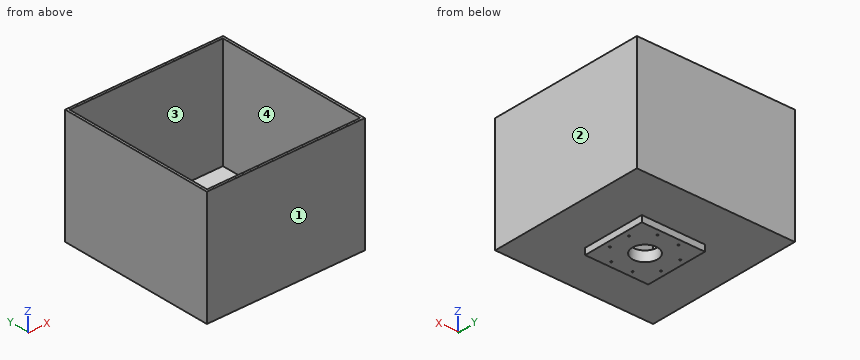
from build123d import *

# Parameters (mm, degrees)
F0_W     = 635
F0_H     = 635
F1_DEPTH = 15.875
F3_DEPTH = 447.675
F4_R     = 50.8
F5_DEPTH = 25.4
F6_W     = 254
F6_H     = 254
F6_R     = 3.4000059
F6_R_2   = 50.8
F7_DEPTH = 25.4


with BuildPart() as f1:
    # F0 (on Top) → F1 (new body)
    with BuildSketch(Plane.XY):
        with Locations((317.5, 317.5)):
            Rectangle(F0_W, F0_H)
    extrude(amount=F1_DEPTH)

    # F2 (on face) → F3 (join)
    with BuildSketch(Plane.XY.offset(15.875)):
        Polygon((0, 635), (0, 625.475), (9.525, 625.475), (625.475, 625.475), (625.475, 635), align=None)
        Polygon((0, 625.475), (0, 0), (9.525, 0), (9.525, 9.525), (9.525, 625.475), align=None)
        Polygon((9.525, 9.525), (9.525, 0), (635, 0), (635, 9.525), (625.475, 9.525), align=None)
        Polygon((625.475, 625.475), (625.475, 9.525), (635, 9.525), (635, 635), (625.475, 635), align=None)
    extrude(amount=F3_DEPTH)

    # F4 (on face) → F5 (cut, symmetric)
    with BuildSketch(Plane(origin=(0, 0, 0), x_dir=(1, 0, 0), z_dir=(0, 0, -1))):
        with Locations((317.5, -317.5)):
            Circle(F4_R)
    extrude(amount=F5_DEPTH, both=True, mode=Mode.SUBTRACT)

    # F6 (on face) → F7 (join)
    with BuildSketch(Plane(origin=(0, 0, 0), x_dir=(1, 0, 0), z_dir=(0, 0, -1))):
        with Locations((317.5, -317.5)):
            Rectangle(F6_W, F6_H)
        with Locations((274.7312995989, -420.7527765535)):
            Circle(F6_R, mode=Mode.SUBTRACT)
        with Locations((214.2472234465, -360.2687004011)):
            Circle(F6_R, mode=Mode.SUBTRACT)
        with Locations((360.2687004011, -420.7527765535)):
            Circle(F6_R, mode=Mode.SUBTRACT)
        with Locations((420.7527765535, -360.2687004011)):
            Circle(F6_R, mode=Mode.SUBTRACT)
        with Locations((214.2472234465, -274.7312995989)):
            Circle(F6_R, mode=Mode.SUBTRACT)
        with BuildLine():
            ThreePointArc((271.3312936989, -214.2472234465), (274.7312995989, -210.8472175465), (278.1313054989, -214.2472234465))
            ThreePointArc((278.1313054989, -214.2472234465), (274.7312995989, -217.6472293465), (271.3312936989, -214.2472234465))
        make_face(mode=Mode.SUBTRACT)
        with Locations((317.5, -317.5)):
            Circle(F6_R_2, mode=Mode.SUBTRACT)
        with Locations((420.7527765535, -274.7312995989)):
            Circle(F6_R, mode=Mode.SUBTRACT)
        with BuildLine():
            ThreePointArc((356.8686945011, -214.2472234465), (360.2687004011, -210.8472175465), (363.6687063011, -214.2472234465))
            ThreePointArc((363.6687063011, -214.2472234465), (360.2687004011, -217.6472293465), (356.8686945011, -214.2472234465))
        make_face(mode=Mode.SUBTRACT)
    extrude(amount=F7_DEPTH)


solid = f1.part
CAD build for the part. Positions are in the model's coordinates, mm. Face numbers are marked on the shaded views. Round coordinates to 2 decimals unless told otherwise and drop trailing zeros. Write each loop counter-clockwise with the first axis right and the second up, starting at its lowest first coordinate (ties: lowest second). Pieces come first, ordered by that corner, then holes. Notation, with made-up numbers: M 12.5,50 L 35.5,50 A7 cw 35.5,56 Z; hole C 39.25,55.5 d4. An arc over 180 degrees is marked long. Put each result on its own line as item: value. Start each with the question number.
1) Saw through at B-B, the plane z = 262. Write the cut outline in (x, y) (3 decimals), and give its area (3 significant figures).
2) Pin check, flat tips, straight feed: pin 1 Ø7.5 at (x, y) = (420, 360.5) entering from -Z; pin 2 Ø1.5 at (x, y) = (236, 336.5) entering from +Z (3 decimals); pin 3 Ø1.5 at (x, y) = (486.5, 170.5) entering from -Z. Stop position of each tip, or through.
3) Saw through at D-D, the plane y = 530. Write the cut outline in (x, z) (3 decimals).
4) Pull direction Y, two halves, no side cores. Call the marked faces 1, 2, 3 and 4: pulls with the +Y half, pulls with the -Y half, needs draft (parallel to the pull), parting line crosses it, or undercut.
5) Drill centre lines: probe 1 along X at (y, z) = (74, 62) (3 decimals); probe 2 along Z at (x, y) = (81, 546.5) (3 decimals). Where is each one in solid material? Low to high. Write a range as [from, to].
6) Saw through at A-A, the plane y = 317.5. Write the cut outline in (x, z) (3 decimals).
Resolved:
1. outline: M 0,0 L 635,0 L 635,635 L 0,635 Z; hole M 9.525,9.525 L 625.475,9.525 L 625.475,625.475 L 9.525,625.475 Z
1. area: 23,800 mm²
2. pin 1: z = -25.4
2. pin 2: z = 15.875
2. pin 3: z = 0
3. outline: M 0,0 L 635,0 L 635,463.55 L 625.475,463.55 L 625.475,15.875 L 9.525,15.875 L 9.525,463.55 L 0,463.55 Z
4. face 1: pulls with the -Y half
4. face 2: needs draft
4. face 3: undercut
4. face 4: undercut
5. probe 1: [0, 9.525], [625.475, 635]
5. probe 2: [0, 15.875]
6. outline: M 0,0 L 190.5,0 L 190.5,-25.4 L 266.7,-25.4 L 266.7,15.875 L 9.525,15.875 L 9.525,463.55 L 0,463.55 Z; M 368.3,-25.4 L 444.5,-25.4 L 444.5,0 L 635,0 L 635,463.55 L 625.475,463.55 L 625.475,15.875 L 368.3,15.875 Z
